```python
from build123d import *

# Parameters (mm, degrees)
SKETCH1_W           = 12.1
SKETCH1_H           = 22.8
SKETCH1_W_2         = 11.9
SKETCH1_H_2         = 22.6
EXTRUDE_THIN1_DEPTH = 7
FILLET1_R           = 0.05


with BuildPart() as part:
    # Sketch1 → Extrude-Thin1 (new body, symmetric)
    with BuildSketch(Plane(origin=(0, 0, 0), x_dir=(1, 0, 0), z_dir=(0, 1, 0))):
        Rectangle(SKETCH1_W, SKETCH1_H)
        Rectangle(SKETCH1_W_2, SKETCH1_H_2, mode=Mode.SUBTRACT)
    extrude(amount=EXTRUDE_THIN1_DEPTH, both=True)

    # Fillet1
    fillet1_edges = [part.edges().sort_by_distance(p)[0] for p in [
        (-6.05, 0, -11.4),
        (6.05, 0, -11.4),
        (6.05, 0, 11.4),
        (-6.05, 0, 11.4),
    ]]
    fillet(fillet1_edges, radius=FILLET1_R)


solid = part.part
```
For this review, take the finished solid that the model builds, in its own axes (mm). Coordinates: 2 decimals unless noted, no trailing zeros. Write each loop counter-clockwise with the first axis right and the second up, starting at its lowest first coordinate (ties: lowest second). Pieces come first, ordered by that corner, then holes. Notation, with made-up numbers: (11.5, -21) - (63.5, -21) arc R23 ccw to (63.5, -5) - close; hole circle Ø7 at (-38, -10). An arc over 180 degrees is marked (long way). Answer in a Markdown table with one row per item. Add a question column.
Q1. For P1, Ø5, axis at x = -3, z = 6.5, coming from the +Y side, flat-tipped, find the tip position at first contact; note if it passes through.
Q2. We need section C-C, the plane y = -5.25. State the section outline as (x, z) points, and give its area (3 significant figures).
Q3. We need section B-B, the plane x = -3. State the section outline as (y, z) points, and give its area (3 significant figures).
Q4. We need section A-A, the plane z = -10. State the section outline as (x, y) points, and give its area (3 significant figures).
Answer list:
| question | item | result |
|---|---|---|
| 1 | P1 | passes through |
| 2 | outline | (-6.05, -11.35) arc R0.05 ccw to (-6, -11.4) - (6, -11.4) arc R0.05 ccw to (6.05, -11.35) - (6.05, 11.35) arc R0.05 ccw to (6, 11.4) - (-6, 11.4) arc R0.05 ccw to (-6.05, 11.35) - close; hole (-5.95, -11.3) - (5.95, -11.3) - (5.95, 11.3) - (-5.95, 11.3) - close |
| 2 | area | 6.94 mm2 |
| 3 | outline | (-7, -11.4) - (7, -11.4) - (7, -11.3) - (-7, -11.3) - close; (-7, 11.3) - (7, 11.3) - (7, 11.4) - (-7, 11.4) - close |
| 3 | area | 2.80 mm2 |
| 4 | outline | (-6.05, -7) - (-5.95, -7) - (-5.95, 7) - (-6.05, 7) - close; (5.95, -7) - (6.05, -7) - (6.05, 7) - (5.95, 7) - close |
| 4 | area | 2.80 mm2 |
